Here's the drawing with two shaded views (mm, measured from the low corner). I have some questions. A direction names the side the tool comes from. Round coordinates to 2 decimals unless told otherwise and drop trailing zeros. Write each loop counter-clockwise with the first axis right and the second up, starting at its lowest first coordinate (ties: lowest second). Pieces come first, ordered by that corner, then holes. Notation, with made-up numbers: (67, 89.25) - (111, 89.25) arc R7 cw to (111, 102.25) - close; hole circle Ø7 at (6, 82). An arc over 180 degrees is marked (long way). Return JSON: item names as keys, results as strings. Group by question number.
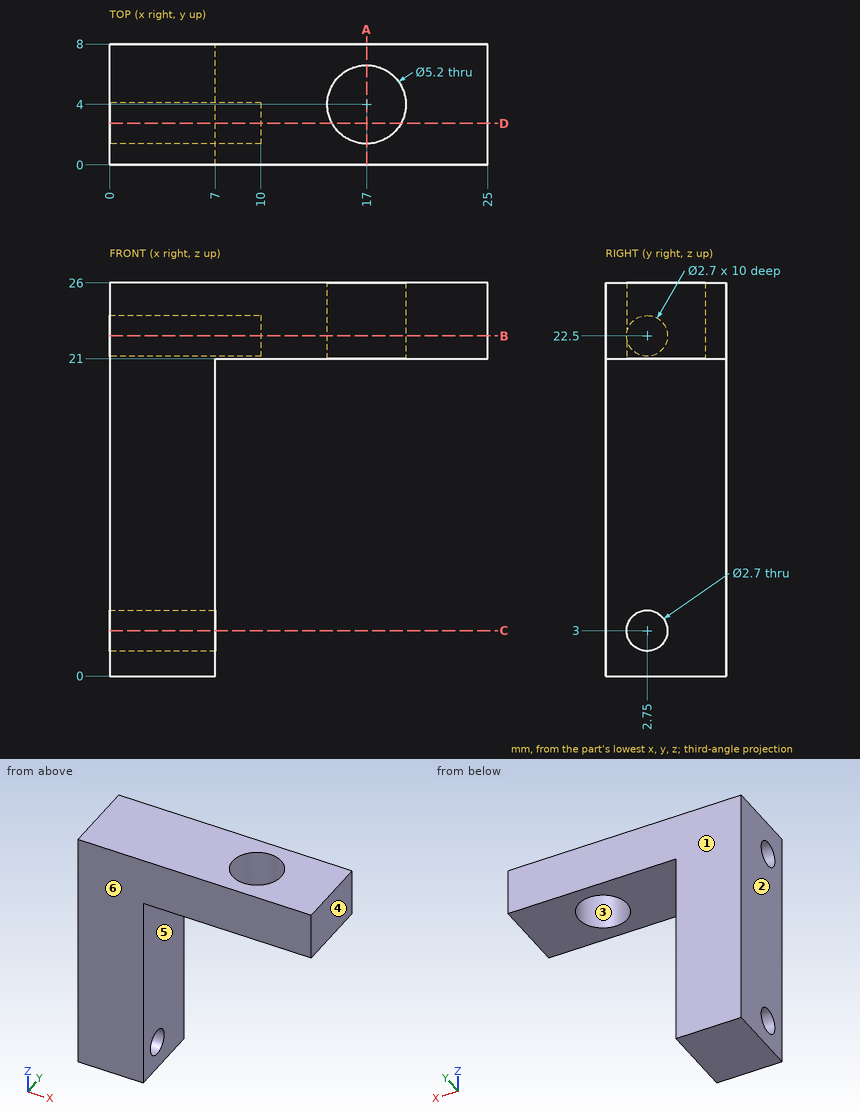
1) Imagine slicing it at B-B (z = 22.5). Please give me the cut outline in (x, y), plus the area to 3 significant figures.
2) Imagine slicing it at A-A (x = 17). Please give me the cut outline in (y, z), plus the area to 3 significant figures.
3) Imagine slicing it at C-C (z = 3). Please give me the cut outline in (x, y).
4) If we mould it in two halves opening along X, with no side actions, what happens to the marked faces 1, 2, 3 and 4? For each: released by +X, released by -X, zero draft, split by the parting line, or undercut.
5) I need wall thicknesses on line 1 along Y through (x, z) = (2.75, 22.5); line 2 along Z through (x, y) = (9.5, 7); line 3 along X through (y, z) = (5.75, 4.75). Which ranges of each line are inside material? Lowest first, please.
6) For the marked faces 5 and 6, which set-ups out of +Z, -Z, +X, -X, +Y, -Y let a thin tool reach every point of the face, with its end or its side?
7) Imagine slicing it at D-D (y = 2.75). Please give me the cut outline in (x, z), plus the area to 3 significant figures.
Results found:
{
 "1": {"outline": "(0, 0) - (25, 0) - (25, 8) - (0, 8) - (0, 4.1) - (10, 4.1) - (10, 1.4) - (0, 1.4) - close; hole circle Ø5.2 at (17, 4)", "area": "152 mm²"},
 "2": {"outline": "(0, 21) - (1.4, 21) - (1.4, 26) - (0, 26) - close; (6.6, 21) - (8, 21) - (8, 26) - (6.6, 26) - close", "area": "14.0 mm²"},
 "3": {"outline": "(0, 0) - (7, 0) - (7, 1.4) - (0, 1.4) - close; (0, 4.1) - (7, 4.1) - (7, 8) - (0, 8) - close"},
 "4": {"face 1": "zero draft", "face 2": "released by -X", "face 3": "undercut", "face 4": "released by +X"},
 "5": {"line 1": "y = 0 to 1.4, 4.1 to 8", "line 2": "z = 21 to 26", "line 3": "x = 0 to 7"},
 "6": {"face 5": "-Z, +X, +Y, -Y", "face 6": "+Z, -Z, +X, -X, -Y"},
 "7": {"outline": "(0, 0) - (7, 0) - (7, 1.65) - (0, 1.65) - close; (0, 4.35) - (7, 4.35) - (7, 21) - (14.72, 21) - (14.72, 26) - (0, 26) - (0, 23.85) - (10, 23.85) - (10, 21.15) - (0, 21.15) - close; (19.28, 21) - (25, 21) - (25, 26) - (19.28, 26) - close", "area": "203 mm²"}
}
